```python
from build123d import *

# Parameters (mm, degrees)
SKETCH1_R                = 30
SKETCH1_R_2              = 7
BOSS_EXTRUDE1_DEPTH      = 10
FILLET1_R                = 10
FILLET2_R                = 20
CUT_EXTRUDE1_DEPTH       = 10
BOSS_EXTRUDE4_DEPTH      = 48
BOSS_EXTRUDE4_DEPTH_BACK = 27
SKETCH3_R                = 10
SKETCH3_R_2              = 7.5


with BuildPart() as part:
    # Sketch1 → Boss-Extrude1 (new, symmetric)
    with BuildSketch(Plane(origin=(0, 0, 0), x_dir=(1, 0, 0), z_dir=(0, 1, 0))):
        with BuildLine():
            Line((27.935473676, -25.760615491), (128.063755469, -9.084385863))
            ThreePointArc((128.063755469, -9.084385863), (155, 0), (128.063755469, 9.084385863))
            Line((128.063755469, 9.084385863), (27.935473676, 25.760615491))
            ThreePointArc((27.935473676, 25.760615491), (-38, 0), (27.935473676, -25.760615491))
        make_face()
        with Locations(Location((0, 0, 0), (0, 0, 270))):
            Circle(SKETCH1_R, mode=Mode.SUBTRACT)
        with Locations(Location((140, 0, 0), (0, 0, 270))):
            Circle(SKETCH1_R_2, mode=Mode.SUBTRACT)
    extrude(amount=BOSS_EXTRUDE1_DEPTH, both=True)

    # Fillet1
    fillet1_edges = [part.edges().sort_by_distance(p)[0] for p in [
        (128.063755469, 0, -9.084385863),
        (128.063755469, 0, 9.084385863),
    ]]
    fillet(fillet1_edges, radius=FILLET1_R)

    # Fillet2
    fillet2_edges = [part.edges().sort_by_distance(p)[0] for p in [
        (27.935473676, 0, -25.760615491),
        (27.935473676, 0, 25.760615491),
    ]]
    fillet(fillet2_edges, radius=FILLET2_R)

    # Sketch2 → Cut-Extrude1 (cut)
    with BuildSketch(Plane(origin=(0, 10, 0), x_dir=(1, 0, 0), z_dir=(0, 1, 0))):
        with BuildLine():
            Line((41.655668603, 18.406663826), (125.154779936, 4.5))
            ThreePointArc((125.154779936, 4.5), (129.654779936, 0), (125.154779936, -4.5))
            Line((125.154779936, -4.5), (41.655668603, -18.406663826))
            ThreePointArc((41.655668603, -18.406663826), (37.03770568, -16.72826346), (36.086072586, -11.907785911))
            ThreePointArc((36.086072586, -11.907785911), (38, 0), (36.086072586, 11.907785911))
            ThreePointArc((36.086072586, 11.907785911), (37.03770568, 16.72826346), (41.655668603, 18.406663826))
        make_face()
    cut_extrude1 = extrude(amount=-CUT_EXTRUDE1_DEPTH, mode=Mode.SUBTRACT)

    # Mirror1: Cut-Extrude1 across plane
    add(cut_extrude1.mirror(Plane.ZX), mode=Mode.SUBTRACT)

    # Sketch3 → Boss-Extrude4 (add, two sides: drawn at the far end of the back side and taken through both)
    with BuildSketch(Plane(origin=(4.107142857, 0, -24.6603199), x_dir=(0.9864127959843347, 0, 0.16428571428571412), z_dir=(-0.16428571428571412, 0, 0.9864127959843348)).offset(-BOSS_EXTRUDE4_DEPTH_BACK)):
        with Locations(Location((113.065732621, 0, 0), (0, 0, 270))):
            Circle(SKETCH3_R)
        with Locations(Location((68.065732621, 0, 0), (0, 0, 180))):
            Circle(SKETCH3_R_2)
    extrude(amount=BOSS_EXTRUDE4_DEPTH + BOSS_EXTRUDE4_DEPTH_BACK)


solid = part.part
```
Geometry: final body of the model. Coordinates: model frame, mm. A direction names the side the tool comes from. Round coordinates to 2 decimals unless told otherwise and drop trailing zeros. Order: outer loops, then holes, each group sorted by start corner. A loop starts at its lowest first (then second) coordinate and runs counter-clockwise, first axis right, second up. Notation, with made-up numbers: M -3.75,61 L 10.25,61 A18 ccw 10.25,69 Z; hole C 55.25,-14 d2. An arc over 180 degrees is marked long. Use one line per item in the form item = value. Start each with the question number.
Q1. Pin query (flat end, axial travel): pin 1 Ø2 at (x, z) = (14, 23.5) entering from -Y; pin 2 Ø8 at (x, y) = (32.5, -1) entering from +Z; pin 3 Ø8 at (y, z) = (7.5, -10) entering from -X; pin 4 Ø10 at (x, y) = (24.5, 3.5) entering from -Z. Return the tip coordinate at first contact, or that it passes through.
Q2. Cut plane C-C (y = -5). Count the separate pieces of the cut face and the enclosed holes in it, and give its area (3 significant figures).
Q3. Material intervals for line 1 (X direction, y = -4.75, z = 26); line 2 (X direction, y = 2.5, z = 20.5); line 3 (Z direction, x = 22.5, y = 6.75), sorted ascending. Write a range as [from, to].
Q4. Cut plane A-A (x = 0). Return loops of the section in (y, z).
Q5. Access query for faces 1 (the face through (38, 0, 0)), 2 (the face through (124.108, -1.528, 4.674)), 3 (the face through (122.841, 7.934, -4.885)), 4 (the face through (37, -10, 0)). Directions: +Z, -Z, +X, -X, +Y, -Y. A direction counts if a zero-diameter tool reaches every point of the face in a straight line with its end or side. Return the directions, or none.
Q6. Cut plane B-B (x = 47.5). Return loops of the section in (y, z), and give its area (3 significant figures).
Q7. Mould query, pull axis X, two halves, no side actions, for faces 5 (the face through (108.66, 2.17, -23.62)), 6 (the face through (28.9, -0.1, 26.3)), 7 (the face through (37, 10, 0)). Classes: +X half, -X half, draft (parallel to the pull), parting line (faces both ways), or undercut.
Geometry results:
q1.pin_1 = through
q1.pin_2 = 26.49
q1.pin_3 = -37.52
q1.pin_4 = -32.62
q2.separate_pieces = 1
q2.enclosed_holes = 5
q2.area = 5,100 mm^2
q3.line_1 = [-27.71, -14.97], [14.97, 29.59], [58.79, 70.56], [101.37, 119.21]
q3.line_2 = [-32, -21.9], [21.9, 72.76], [101.39, 121.02]
q3.line_3 = [-30.62, -19.84], [19.84, 30.62]
q4.outline = M -10,-38 L 10,-38 L 10,-30 L -10,-30 Z; M -10,30 L 10,30 L 10,38 L -10,38 Z
q5.face_1 = +Y, -Y
q5.face_2 = none
q5.face_3 = +Y
q5.face_4 = +Z, -Z, +X, -X, -Y
q6.outline = M -10,-22.5 L 10,-22.5 L 10,-17.43 L -10,-17.43 Z; M -10,17.43 L 10,17.43 L 10,22.5 L -10,22.5 Z
q6.area = 203 mm^2
q7.face_5 = undercut
q7.face_6 = undercut
q7.face_7 = draft
